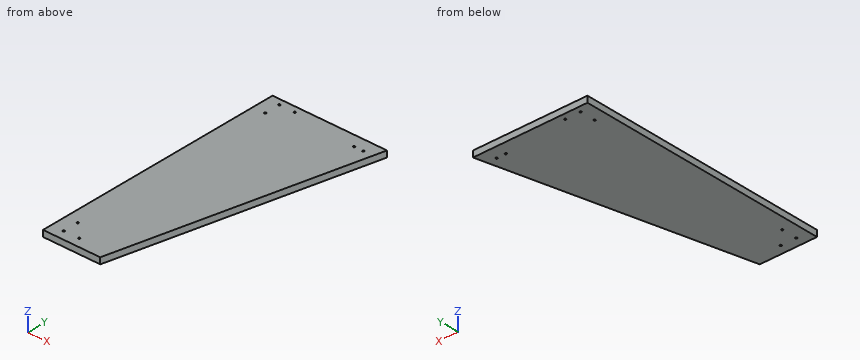
```python
from build123d import *

# Parameters (mm, degrees)
EXTRUDE_1_DEPTH     = 10
SKETCH_2_R          = 1.5
CUT_EXTRUDE_1_DEPTH = 10
SKETCH_3_R          = 1.5
CUT_EXTRUDE_2_DEPTH = 10


with BuildPart() as part:
    # 草图1 → 凸台-拉伸1 (new body)
    with BuildSketch(Plane.XY):
        Polygon((185, 0), (0, 0), (0, -400), (0, -410), (92.5, -410), align=None)
    extrude(amount=EXTRUDE_1_DEPTH)

    # 草图2 → 切除-拉伸1 (cut)
    with BuildSketch(Plane.XY.offset(10)):
        with Locations((20, -35)):
            Circle(SKETCH_2_R)
        with Locations((45, -10)):
            Circle(SKETCH_2_R)
        with Locations((20, -10)):
            Circle(SKETCH_2_R)
        with Locations((45, -395)):
            Circle(SKETCH_2_R)
        with Locations((20, -395)):
            Circle(SKETCH_2_R)
        with Locations((20, -370)):
            Circle(SKETCH_2_R)
    extrude(amount=-CUT_EXTRUDE_1_DEPTH, mode=Mode.SUBTRACT)

    # 草图3 → 切除-拉伸2 (cut)
    with BuildSketch(Plane(origin=(0, 0, 0), x_dir=(-1, 0, 0), z_dir=(0, 0, -1))):
        with Locations((-165, -20)):
            Circle(SKETCH_3_R)
        with Locations((-150, -20)):
            Circle(SKETCH_3_R)
    extrude(amount=-CUT_EXTRUDE_2_DEPTH, mode=Mode.SUBTRACT)


solid = part.part
```
Input: part model. Units: mm. Frame: model coordinates. Round coordinates to 2 decimals unless told otherwise and drop trailing zeros. Loops run counter-clockwise (first coordinate to the right, second up) from the corner with the lowest first, then second, coordinate; pieces in that order, holes last. Notation, with made-up numbers: (67, -23.5) -> (121, -23.5) arc R11 cw to (121, -3.5) -> close; hole circle Ø11 at (66.5, -6). An arc over 180 degrees is marked (long way). One line per item, written item: value.
(1) Material intervals for line 1 (Y direction, x = 45, z = 4.25); line 2 (Y direction, x = 20, z = 6.75); line 3 (X direction, y = -395, z = 5), sorted ascending. Write a range as [from, to].
Geometry check:
line 1: [-410, -396.5], [-393.5, -11.5], [-8.5, 0]
line 2: [-410, -396.5], [-393.5, -371.5], [-368.5, -36.5], [-33.5, -11.5], [-8.5, 0]
line 3: [0, 18.5], [21.5, 43.5], [46.5, 95.88]
(2) Section B-B (y = -364.5). Return the cut outline in (x, z).
Geometry check:
outline: (0, 0) -> (102.77, 0) -> (102.77, 10) -> (0, 10) -> close
(3) Section C-C (x = 137). Return the cut outline in (y, z), plus the area to 3 significant figures.
Geometry check:
outline: (-212.76, 0) -> (0, 0) -> (0, 10) -> (-212.76, 10) -> close
area: 2,130 mm2
(4) Section A-A (z = 1.75). Give the number of separate pieces and of enclosed holes in the cut face, plus the area to 3 significant figures.
Geometry check:
separate pieces: 1
enclosed holes: 8
area: 56,800 mm2
